from build123d import *

# Parameters (mm, degrees)
F1_DEPTH = 32
F2_R     = 1
F3_R     = 5
F4_SIZE  = 2
F5_SIZE  = 1
F7_DEPTH = 4.5


with BuildPart() as f1:
    # F0 (on Front) → F1 (new body)
    with BuildSketch(Plane.XZ):
        Polygon((0, 0), (0, 90), (-4.5, 90), (-4.5, 4.5), (-28, 4.5), (-28, 0), align=None)
    extrude(amount=F1_DEPTH)

    # F2
    f2_edges = [f1.edges().sort_by_distance(p)[0] for p in [
        (-4.5, -16, 4.5),
    ]]
    fillet(f2_edges, radius=F2_R)

    # F3
    f3_edges = [f1.edges().sort_by_distance(p)[0] for p in [
        (0, -16, 0),
    ]]
    fillet(f3_edges, radius=F3_R)

    # F4
    f4_edges = [f1.edges().sort_by_distance(p)[0] for p in [
        (0, -16, 90),
    ]]
    chamfer(f4_edges, length=F4_SIZE)

    # F5
    f5_edges = [f1.edges().sort_by_distance(p)[0] for p in [
        (-28, -32, 2.25),
        (-28, 0, 2.25),
    ]]
    chamfer(f5_edges, length=F5_SIZE)

    # F6 (on face) → F7 (cut)
    with BuildSketch(Plane.XY.offset(4.5)):
        with BuildLine():
            ThreePointArc((-15, -10.5), (-11.5, -7), (-15, -3.5))
            Line((-15, -3.5), (-21, -3.5))
            ThreePointArc((-21, -3.5), (-24.5, -7), (-21, -10.5))
            Line((-21, -10.5), (-15, -10.5))
        make_face()
        with BuildLine():
            ThreePointArc((-15, -28.5), (-11.5, -25), (-15, -21.5))
            Line((-15, -21.5), (-21, -21.5))
            ThreePointArc((-21, -21.5), (-24.5, -25), (-21, -28.5))
            Line((-21, -28.5), (-15, -28.5))
        make_face()
    extrude(amount=-F7_DEPTH, mode=Mode.SUBTRACT)


solid = f1.part
Verification items for the finished model (mm, model axes). A direction names the side the tool comes from. Round coordinates to 2 decimals unless told otherwise and drop trailing zeros. Order: outer loops, then holes, each group sorted by start corner. A loop starts at its lowest first (then second) coordinate and runs counter-clockwise, first axis right, second up. Notation, with made-up numbers: (60.5, 23) -> (90.5, 23) arc R19 ccw to (90.5, 38) -> close; hole circle Ø7 at (-34.5, 42). An arc over 180 degrees is marked (long way). Put each result on its own line as item: value.
1) Section check A-A (y = -5.5). Record the cut outline in (x, z).
Final values:
outline: (-28, 0) -> (-24.16, 0) -> (-24.16, 4.5) -> (-28, 4.5) -> close; (-11.84, 0) -> (-5, 0) arc R5 ccw to (0, 5) -> (0, 88) -> (-2, 90) -> (-4.5, 90) -> (-4.5, 5.5) arc R1 cw to (-5.5, 4.5) -> (-11.84, 4.5) -> close
2) Section check B-B (y = -30). Record the cut outline in (x, z).
Final values:
outline: (-28, 0) -> (-5, 0) arc R5 ccw to (0, 5) -> (0, 88) -> (-2, 90) -> (-4.5, 90) -> (-4.5, 5.5) arc R1 cw to (-5.5, 4.5) -> (-28, 4.5) -> close
3) Material ranges on line 1 (Z direction, x = -25.25, y = -12); line 2 (X direction, y = -5.5, z = 13); line 3 (Z direction, x = -3.75, y = -19.5), recorded low to high.
Final values:
line 1: z = 0 to 4.5
line 2: x = -4.5 to 0
line 3: z = 0.16 to 90
4) Mould release check, pull along X, two halves, no side actions. Record for faces 1 (the flat face through (-17, -16, 4.5)), 2 (the flat face through (-28, -16, 2)), 3 (the flat face through (-18, -28.5, 2)): +X half, -X half, draft (parallel to the pull), parting line (faces both ways), or undercut.
Final values:
face 1: draft
face 2: -X half
face 3: undercut
5) Section check C-C (z = 51). Record the cut outline in (x, y), then the cut area to 3 significant figures.
Final values:
outline: (-4.5, -32) -> (0, -32) -> (0, 0) -> (-4.5, 0) -> close
area: 144 mm^2
6) Set-up check for faces 4 (the flat face through (-3, -16, 90)), 5 (the flat face through (-4.5, -16, 48)), 6 (the flat face through (-18, -10.5, 2)): record each of +Z, -Z, +X, -X, +Y, -Y from which the full face is reachable in a straight line by a thin tool's end or side.
Final values:
face 4: +Z, +X, -X, +Y, -Y
face 5: +Z, -X, +Y, -Y
face 6: +Z, -Z
7) Section check D-D (y = -25). Record the cut outline in (x, z), then the cut area to 3 significant figures.
Final values:
outline: (-28, 0) -> (-24.5, 0) -> (-24.5, 4.5) -> (-28, 4.5) -> close; (-11.5, 0) -> (-5, 0) arc R5 ccw to (0, 5) -> (0, 88) -> (-2, 90) -> (-4.5, 90) -> (-4.5, 5.5) arc R1 cw to (-5.5, 4.5) -> (-11.5, 4.5) -> close
area: 445 mm^2
8) Depth check by flat-ended pin: pin 1 (12 mm diameter, centred on y = -25, z = 73.5, fed in from -X); pin 2 (1 mm diameter, centred on x = -10, y = -16, fed in from +Z). Enter the tip coordinate at first touch or a pass-through.
Final values:
pin 1: stops at x = -4.5
pin 2: stops at z = 4.5
